Geometry check sheet. Reference: drawing and pictorial views, mm from the part's lowest x, y, z. A direction names the side the tool comes from. Coordinates: 2 decimals unless noted, no trailing zeros. Loops run counter-clockwise (first coordinate to the right, second up) from the corner with the lowest first, then second, coordinate; pieces in that order, holes last. Notation, with made-up numbers: (-11, 23) -> (43, 23) arc R18 cw to (43, 42) -> close; hole circle Ø9 at (62, 63.25). An arc over 180 degrees is marked (long way). Use one line per item in the form item = value.
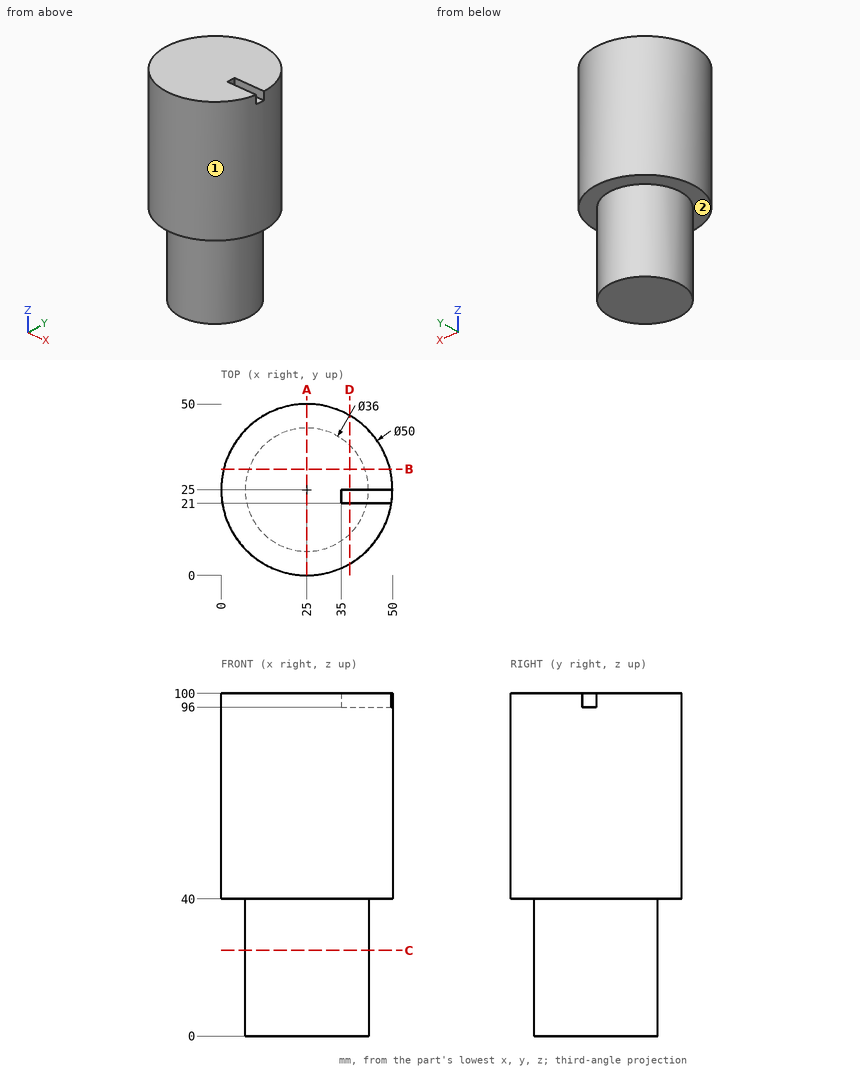
(1) Go/stop test with flat-tipped pins: P1, Ø1.2, axis at x = 41.5, z = 97.5, coming from the -Y side; P2, Ø2, axis at y = 21.5, z = 60, coming from the +X side; P3, Ø6, axis at x = 31.5, z = 15, coming from the -Y side. Record where each tip stops, or that it passes through.
Established:
P1 = 5.71
P2 = 49.87
P3 = 7.34
(2) Section check C-C, the plane z = 25. Record the boundary of the cut face in (x, y), plus the area to 3 significant figures.
Established:
outline = circle Ø36 at (25, 25)
area = 1,020 mm²
(3) Tool access check on the marked faces 1 and 2. Record the directions out of +Z, -Z, +X, -X, +Y, -Y that give a thin tool (end or side, any length) a straight path to the whole face; none if there is none.
Established:
face_1 = +Z, -Z
face_2 = -Z
(4) Section check B-B, the plane y = 31. Record the boundary of the cut face in (x, z).
Established:
outline = (0.73, 40) -> (8.03, 40) -> (8.03, 0) -> (41.97, 0) -> (41.97, 40) -> (49.27, 40) -> (49.27, 100) -> (0.73, 100) -> close
(5) Scan lines: line 1 along Z through (x, y) = (5.5, 26); line 2 along Y through (x, z) = (24.5, 84) (3 decimals). Record each from-to range of solid material in increasing order.
Established:
line_1 = 40 to 100
line_2 = 0.005 to 49.995
(6) Section check D-D, the plane x = 37.5. Record the boundary of the cut face in (y, z), plus the area to 3 significant figures.
Established:
outline = (3.35, 40) -> (12.05, 40) -> (12.05, 0) -> (37.95, 0) -> (37.95, 40) -> (46.65, 40) -> (46.65, 100) -> (25, 100) -> (25, 96) -> (21, 96) -> (21, 100) -> (3.35, 100) -> close
area = 3,620 mm²
(7) Section check A-A, the plane x = 25. Record the boundary of the cut face in (y, z), plus the area to 3 significant figures.
Established:
outline = (0, 40) -> (7, 40) -> (7, 0) -> (43, 0) -> (43, 40) -> (50, 40) -> (50, 100) -> (0, 100) -> close
area = 4,440 mm²
